Read the model definition and answer for the solid it produces. Units are mm, in the model's axes. A direction names the side the tool comes from. Give positions to 0.01 mm unless a question says otherwise; leave off trailing zeros. Write each loop counter-clockwise with the first axis right and the second up, starting at its lowest first coordinate (ties: lowest second). Pieces come first, ordered by that corner, then holes. Notation, with made-up numbers: M -24,7 L -15,7 A22 ccw -15,19 Z; hole C 2.5,-16 d7. An arc over 180 degrees is marked long. Write each question's results on one line, items separated by ' | '. Start each with the question number.
Autodesk Inventor part; units mm, degrees
ref_plane "YZ Plane" through (0, 0, 0) normal (1, 0, 0) x (0, 1, 0)
ref_plane "XZ Plane" through (0, 0, 0) normal (0, 1, 0) x (-1, 0, 0)
ref_plane "XY Plane" through (0, 0, 0) normal (0, 0, 1) x (1, 0, 0)
sketch "Sketch1" plane through (0, 0, 0) normal (0, 0, 1) x (1, 0, 0)
  line L0 (0, 0) -> (137, 0)
  line L1 (137, 0) -> (137, 35)
  line L2 (137, 35) -> (0, 35)
  line L3 (0, 35) -> (0, 0)
  line L4 (141, 30.1) -> (137, 30.1)
  line L5 (137, 30.1) -> (137, 9.9)
  line L6 (137, 9.9) -> (141, 9.9)
  line L7 (141, 9.9) -> (141, 30.1)
  line L8 (141, 30.1) -> (137, 9.9) construction
  line L9 (137, 30.1) -> (141, 9.9) construction
  line L10 (-4, 30.1) -> (0, 30.1)
  line L11 (0, 30.1) -> (0, 9.9)
  line L12 (0, 9.9) -> (-4, 9.9)
  line L13 (-4, 9.9) -> (-4, 30.1)
  line L14 (-4, 30.1) -> (0, 9.9) construction
  line L15 (0, 30.1) -> (-4, 9.9) construction
  point P0 (139, 20)
  point P1 (-2, 20)
  point P2 (0, 30.1)
  point P3 (0, 30.1)
  point P4 (137, 30.1)
  point P5 (100, 25)
  point P6 (0, 25)
  dimension "d0" = 4
  dimension "d1" = 4
  dimension "d2" = 137
  dimension "d3" = 35
  dimension "d4" = 20.2
  dimension "d5" = 9.9
extrude "Extrusion1" add sketch "Sketch1" along normal blind 3
properties part number "Battary_holder_part2"
Item 1: A straight line is drawn through the part: line 1 (X direction, y = 32.5, z = 2.15). Find the intervals that lie inside material, in ascending order.
Item 2: Section B-B, the plane y = 4 is taken. Determine the outline of the cut face in (x, z), then the cut area to 3 significant figures.
Item 3: Given P1, Ø1.5, axis at x = -2, z = 2, coming from the -Y side; P2, Ø0.9, axis at y = 4, z = 1, coming from the -X side; P3, Ø1.5, axis at y = 6.5, z = 1, coming from the +X side, each flat-ended and moving along its own axis, determine where each tip first touches the part or whether it passes through.
Item 4: Section A-A, the plane z = 1.2 is taken. Determine the outline of the cut face in (x, y).
Item 5: For faces 1 (the flat face through (0, 5, 1)), 2 (the flat face through (0, 33, 1)), 3 (the flat face through (137, 5, 1)), 4 (the flat face through (139, 30.1, 1)), determine the directions among +Z, -Z, +X, -X, +Y, -Y from which every point of the face is accessible in a straight line to the end or side of a thin tool.
Worked out:
1) line 1: x = 0 to 137
2) outline: M 0,0 L 137,0 L 137,3 L 0,3 Z | area: 411 mm²
3) P1: stops at y = 9.9 | P2: stops at x = 0 | P3: stops at x = 137
4) outline: M -4,9.9 L 0,9.9 L 0,0 L 137,0 L 137,9.9 L 141,9.9 L 141,30.1 L 137,30.1 L 137,35 L 0,35 L 0,30.1 L -4,30.1 Z
5) face 1: +Z, -Z, -X, -Y | face 2: +Z, -Z, -X, +Y | face 3: +Z, -Z, +X, -Y | face 4: +Z, -Z, +X, +Y
